Autodesk Inventor part; units mm, degrees
ref_plane "YZ Plane" through (0, 0, 0) normal (1, 0, 0) x (0, 1, 0)
ref_plane "XZ Plane" through (0, 0, 0) normal (0, 1, 0) x (-1, 0, 0)
ref_plane "XY Plane" through (0, 0, 0) normal (0, 0, 1) x (1, 0, 0)
sketch "Sketch1" plane through (0, 0, 0) normal (0, 0, 1) x (1, 0, 0)
  line L0 (10.7104, 9.7791) -> (45.7104, 9.7791)
  line L1 (45.7104, 9.7791) -> (45.7104, 24.7791)
  line L2 (10.7104, 9.7791) -> (10.7104, 24.7791)
  line L3 (5.7104, 24.7791) -> (5.7104, 4.7791)
  line L4 (5.7104, 4.7791) -> (50.7104, 4.7791)
  line L5 (50.7104, 4.7791) -> (50.7104, 24.7791)
  line L6 (5.7104, 24.7791) -> (10.7104, 24.7791)
  line L7 (45.7104, 24.7791) -> (50.7104, 24.7791)
  point P0 (0, 0)
  point P1 (28.2104, 9.7791)
  dimension "d0" = 35
  dimension "d1" = 15
  dimension "d2" = 15
  dimension "d29" = 5
extrude "Extrusion1" add sketch "Sketch1" along normal blind 100
sketch "Sketch3" plane through (10.7104, 9.7791, 0) normal (0, 1, 0) x (1, 0, 0)
  line L0 (-5, -100) -> (40, -100)
  line L1 (-5, 0) -> (-5, -100)
  line L2 (17.5, -100) -> (37.1919, -100) construction
  line L3 (-5, -85.7353) -> (-5, -100)
  line L4 (-5, -100) -> (17.5, -100)
  line L5 (40, 0) -> (40, -100)
  line L6 (17.5, -100) -> (37.1919, -100) construction
  line L7 (40, -85.7353) -> (40, -100)
  line L8 (40, -100) -> (17.5, -100)
  line L9 (40, 0) -> (40, -100)
  line L10 (17.5, -100) -> (-5, -66.9281)
  line L11 (17.5, -100) -> (40, -66.9281)
  point P0 (-10.7104, 0)
  point P1 (-5, -77.7514)
  point P2 (40, -66.9281)
  dimension "d20" = 40
  dimension "d23" = 40
  dimension "d27" = 55.771
  dimension "d28" = 68.458
extrude "Extrusion5" cut sketch "Sketch3" along normal through all both and the other way through all
sketch "Sketch4" plane through (50.7104, 4.7791, 0) normal (1, 0, 0) x (0, 0, -1)
  line L0 (0, 20) -> (-74.2774, 20)
  line L1 (0, 20) -> (-4, 20)
  line L2 (-4, 20) -> (-4, 5)
  line L3 (0, 5) -> (-74.2774, 5)
  line L4 (0, 20) -> (0, 5)
  line L5 (0, 5) -> (0, 20)
  line L6 (0, 20) -> (0, 5)
  line L7 (-4, 5) -> (0, 5)
  point P0 (0, -4.7791)
  dimension "d24" = 4
extrude "Extrusion6" cut sketch "Sketch4" against normal through all
equation "\"d23\" = d20"
equation "\"BendRadius\" = Thickness"
equation "\"BendReliefWidth\" = Thickness"
equation "\"BendReliefDepth\" = 0.5 * Thickness"
equation "\"CornerReliefSize\" = 4 * Thickness"
equation "\"MinimumRemnant\" = 2 * Thickness"
equation "\"TransitionRadius\" = BendRadius"
equation "\"JacobiRadiusSize\" = BendRadius"
equation "\"GapSize\" = Thickness"
properties part number "middleslide"
The listing builds one solid part. Answer for the finished solid, in the listing's coordinates (mm). A direction names the side the tool comes from. Coordinates: 2 decimals unless noted, no trailing zeros. Loops run counter-clockwise (first coordinate to the right, second up) from the corner with the lowest first, then second, coordinate; pieces in that order, holes last. Notation, with made-up numbers: (79.25, 67) - (127.25, 67) arc R23 ccw to (127.25, 90) - close; hole circle Ø10 at (82.25, 44.25). An arc over 180 degrees is marked (long way). Use a Markdown table: item, result. Add a question column.
1) The part is cut by section D-D, the plane x = 20. Give the vertices of the cut face in (y, z).
2) The mould has two halves that part along X. Classify faces 4 (the flat face through (10.71, 17, 39)), 5 (the flat face through (44.3, 7.97, 76.35)), 6 (the flat face through (8, 24.779, 39)): released by +X, released by -X, zero draft, split by the parting line, or undercut.
3) The part is cut by section B-B, the plane z = 29.5. Give the vertices of the cut face in (x, y), and give its area (3 significant figures).
4) The part is cut by section C-C, the plane y = 8. Give the vertices of the cut face in (x, z), and give its area (3 significant figures).
5) Find the intervals of material crossed by line 1 (X direction, y = 11.5, z = 7); line 2 (Y direction, x = 29.5, z = 11); line 3 (X direction, y = 17, z = 68.5), in increasing order.
6) The part is cut by section A-A, the plane y = 15.25. Give the vertices of the cut face in (x, z).
7) For faces 1 (the flat face through (5.71, 15, 33)), 2 (the flat face through (8, 17, 4)), 3 (the flat face through (45.71, 17, 39)), determine the directions among +Z, -Z, +X, -X, +Y, -Y from which every point of the face is accessible in a straight line to the end or side of a thin tool.
8) Given pin 1 (1 mm diameter, centred on y = 18, z = 69.5, fed in from -X); pin 2 (1 mm diameter, centred on x = 11, y = 14.5, fed in from -Z); pin 3 (13.5 mm diameter, centred on x = 28, z = 44, fed in from +Y), each flat-ended and moving along its own axis, determine where each tip first touches the part or whether it passes through.
Here are the results:
| question | item | result |
|---|---|---|
| 1 | outline | (4.78, 0) - (9.78, 0) - (9.78, 87.93) - (4.78, 87.93) - close |
| 2 | face 4 | undercut |
| 2 | face 5 | released by +X |
| 2 | face 6 | zero draft |
| 3 | outline | (5.71, 4.78) - (50.71, 4.78) - (50.71, 24.78) - (45.71, 24.78) - (45.71, 9.78) - (10.71, 9.78) - (10.71, 24.78) - (5.71, 24.78) - close |
| 3 | area | 375 mm^2 |
| 4 | outline | (5.71, 0) - (50.71, 0) - (50.71, 66.93) - (28.21, 100) - (5.71, 66.93) - close |
| 4 | area | 3,760 mm^2 |
| 5 | line 1 | x = 5.71 to 10.71, 45.71 to 50.71 |
| 5 | line 2 | y = 4.78 to 9.78 |
| 5 | line 3 | x = 6.78 to 10.71, 45.71 to 49.64 |
| 6 | outline | (5.71, 4) - (10.71, 4) - (10.71, 74.28) - (5.71, 66.93) - close; (45.71, 4) - (50.71, 4) - (50.71, 66.93) - (45.71, 74.28) - close |
| 7 | face 1 | +Z, -Z, -X, +Y, -Y |
| 7 | face 2 | -Z, +X, -X, +Y |
| 7 | face 3 | +Z, -Z, +Y |
| 8 | pin 1 | stops at x = 7.12 |
| 8 | pin 2 | stops at z = 4 |
| 8 | pin 3 | stops at y = 9.78 |
